```python
from build123d import *

# Parameters (mm, degrees)
SKETCH_W     = 15
SKETCH_H     = 15
PAD_DEPTH    = 2
PAD001_DEPTH = 5
SKETCH002_R  = 2.5
POCKET_DEPTH = 5


with BuildPart() as part:
    # Sketch → Pad (new body)
    with BuildSketch(Plane.XY):
        Rectangle(SKETCH_W, SKETCH_H)
    extrude(amount=PAD_DEPTH)

    # Sketch001 (on Face6 of Pad) → Pad001 (join)
    with BuildSketch(Plane.XY.offset(2)):
        Polygon((-7.5, 7.5), (7.5, 7.5), (7.5, -7.5), (5.5, -7.5), (5.5, 5.5), (-7.5, 5.5), align=None)
    extrude(amount=PAD001_DEPTH)

    # Sketch002 (on Face3 of Pad001) → Pocket (cut)
    with BuildSketch(Plane.XY.offset(2)):
        with Locations((2.75, 2.75)):
            Circle(SKETCH002_R)
    extrude(amount=-POCKET_DEPTH, mode=Mode.SUBTRACT)


solid = part.part
```
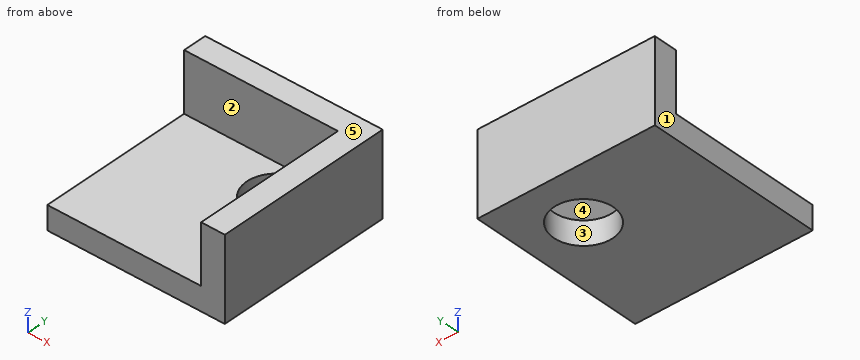
The listing builds one solid part. Answer for the finished solid, in the listing's coordinates (mm). Face numbers are marked on the shaded views. A direction names the side the tool comes from. Round coordinates to 2 decimals unless told otherwise and drop trailing zeros. Loops run counter-clockwise (first coordinate to the right, second up) from the corner with the lowest first, then second, coordinate; pieces in that order, holes last. Notation, with made-up numbers: (43.5, 66.5) - (58.5, 66.5) arc R16 ccw to (58.5, 81.5) - close; hole circle Ø5 at (70, 11.5). An arc over 180 degrees is marked (long way). Return JSON: item names as keys, results as strings. Group by question number.
1. This flat-tipped pin is pushed along its axis until it touches: P1, Ø1, axis at x = -3, y = 0, coming from the +Z side. Where does it stop, or does it pass through?
2. The mould has two halves that part along X. Classify the marked faces 3, 4 and 5: pulls with the +X half, pulls with the -X half, needs draft (parallel to the pull), parting line crosses it, or undercut.
3. Which of the six approach directions +Z, -Z, +X, -X, +Y, -Y give full straight-line access (tool end or side, diameter ignored) to the marked faces 1 and 2?
4. Consider probe 1 along Y at (x, z) = (2.75, 1.1); probe 2 along Z at (x, y) = (1.5, -4.5); probe 3 along X at (y, z) = (-0.5, 4.75). Determine where each line is inside the solid, lowest interval first.
5. The part is cut by section D-D on x = -3. Determine the outline of the cut face in (y, z), then the cut area to 3 significant figures.
6. The part is cut by section C-C on z = 0.75. Determine the outline of the cut face in (x, y), then the cut area to 3 significant figures.
7. The part is cut by section A-A on x = 2.75. Determine the outline of the cut face in (y, z).
Resolved:
{
 "1": {"P1": "stops at z = 2"},
 "2": {"face 3": "undercut", "face 4": "pulls with the -X half", "face 5": "needs draft"},
 "3": {"face 1": "+Z, -Z, -X, +Y, -Y", "face 2": "+Z, -X, -Y"},
 "4": {"probe 1": "y = -7.5 to 0.25, 5.25 to 7.5", "probe 2": "z = 0 to 2", "probe 3": "x = 5.5 to 7.5"},
 "5": {"outline": "(-7.5, 0) - (7.5, 0) - (7.5, 7) - (5.5, 7) - (5.5, 2) - (-7.5, 2) - close", "area": "40.0 mm²"},
 "6": {"outline": "(-7.5, -7.5) - (7.5, -7.5) - (7.5, 7.5) - (-7.5, 7.5) - close; hole circle Ø5 at (2.75, 2.75)", "area": "205 mm²"},
 "7": {"outline": "(-7.5, 0) - (0.25, 0) - (0.25, 2) - (-7.5, 2) - close; (5.25, 0) - (7.5, 0) - (7.5, 7) - (5.5, 7) - (5.5, 2) - (5.25, 2) - close"}
}
